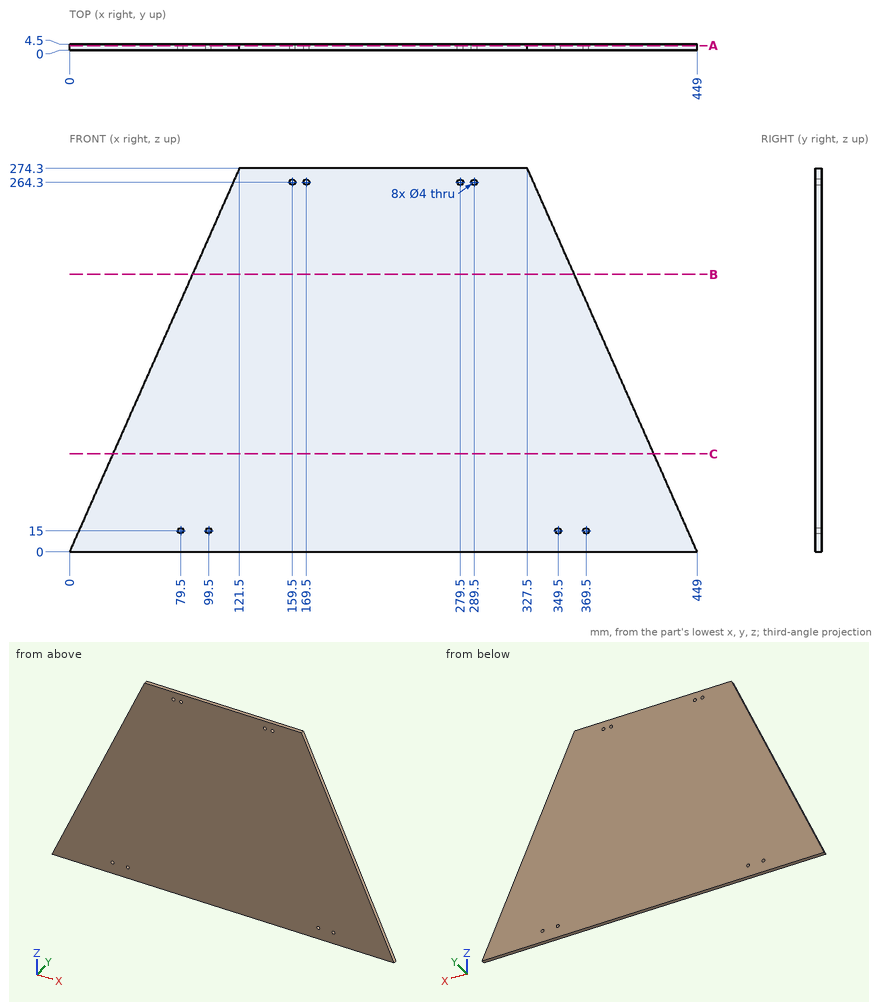
Check sheet for the drawn part. Datum: minimum x, y, z corner. Units: mm. Give positions to 0.01 mm unless a question says otherwise; leave off trailing zeros. Order: outer loops, then holes, each group sorted by start corner. A loop starts at its lowest first (then second) coordinate and runs counter-clockwise, first axis right, second up. Notation, with made-up numbers: (-3.75, 63.25) - (39.25, 63.25) arc R25 cw to (39.25, 97.25) - close; hole circle Ø10 at (-27.75, 39). An arc over 180 degrees is marked (long way). Write item = value, one per line. Start each with the question number.
1) Section check B-B (z = 198.5). Enter the section's corners in (x, y), then the cut area to 3 significant figures.
2) Gauge pin test, flat ends, axial feed: pin 1 Ø6.5 at (x, z) = (349.5, 15) entering from -Y; pin 2 Ø2 at (y, z) = (3, 222) entering from -X; pin 3 Ø2 at (y, z) = (3.5, 119.5) entering from -X; pin 4 Ø1 at (y, z) = (2.5, 164.5) entering from +X. Record the tip position at first contact, or that the pin passes through.
3) Section check A-A (y = 3.4). Count the separate pieces of the cut face and the enclosed holes in it, then the cut area to 3 significant figures.
4) Section check C-C (z = 70). Enter the section's corners in (x, y).
5) Scan lines: L1, parallel to Z at x = 279.5, y = 3.2; L2, parallel to X at y = 1.05, z = 15; L3, parallel to X at y = 3.35, z = 264.3. Record each from-to range of solid material in increasing order.
Geometry check:
q1.outline = (87.92, 0) - (361.08, 0) - (361.08, 4.5) - (87.92, 4.5) - close
q1.area = 1,230 mm2
q2.pin_1 = 0
q2.pin_2 = 97.89
q2.pin_3 = 52.49
q2.pin_4 = 376.36
q3.separate_pieces = 1
q3.enclosed_holes = 8
q3.area = 89,700 mm2
q4.outline = (31.01, 0) - (417.99, 0) - (417.99, 4.5) - (31.01, 4.5) - close
q5.L1 = 0 to 262.3, 266.3 to 274.3
q5.L2 = 6.64 to 77.5, 81.5 to 97.5, 101.5 to 347.5, 351.5 to 367.5, 371.5 to 442.36
q5.L3 = 117.07 to 157.5, 161.5 to 167.5, 171.5 to 277.5, 281.5 to 287.5, 291.5 to 331.93
